```python
from build123d import *

# Parameters (mm, degrees)
BOSS_EXTRU_1_DEPTH      = 5
BOSS_EXTRU_2_DEPTH      = 80
ESQUISSE5_R             = 1.5
ENL_V_MAT_EXTRU_1_DEPTH = 85


with BuildPart() as part:
    # Esquisse1 → Boss.-Extru.1 (new body)
    with BuildSketch(Plane.XY):
        Polygon((90, 47.5), (80, 47.5), (80, 27.5), (90, 27.5), (90, 0), (80, 0), (80, 5), (60, 5), (60, 0), (30, 0), (30, 5), (10, 5), (10, 0), (0, 0), (0, 75), (10, 75), (10, 70), (30, 70), (30, 75), (60, 75), (60, 70), (80, 70), (80, 75), (90, 75), align=None)
    extrude(amount=BOSS_EXTRU_1_DEPTH)

    # Esquisse3 → Boss.-Extru.2 (add)
    with BuildSketch(Plane.ZY):
        Polygon((5, 18), (15, 18), (15, 5.25), (10, 5.25), (10, 13), (5, 13), align=None)
        Polygon((5, 62), (5, 57), (15, 57), (15, 69.75), (10, 69.75), (10, 62), align=None)
    extrude(amount=-BOSS_EXTRU_2_DEPTH)

    # Esquisse5 → Enlèv. mat.-Extru.1 (cut)
    with BuildSketch(Plane.ZY):
        with Locations((2.5, 2.5)):
            Circle(ESQUISSE5_R)
        with Locations((2.5, 72.5)):
            Circle(ESQUISSE5_R)
    extrude(amount=-ENL_V_MAT_EXTRU_1_DEPTH, mode=Mode.SUBTRACT)


solid = part.part
```
Geometry check sheet. Reference: the model listing, model coordinates, mm. A direction names the side the tool comes from. Give positions to 0.01 mm unless a question says otherwise; leave off trailing zeros. Loops run counter-clockwise (first coordinate to the right, second up) from the corner with the lowest first, then second, coordinate; pieces in that order, holes last. Notation, with made-up numbers: M 63,-27.5 L 96,-27.5 A22 cw 96,7.5 Z; hole C 28.5,72.25 d6. An arc over 180 degrees is marked long. Write item = value, one per line. Start each with the question number.
1. Draft check along Z on faces 6 (the face through (39, 63, 15)), 7 (the face through (85, 73, 2)), 8 (the face through (0, 37, 4)). Enter one of: +Z half, -Z half, draft (parallel to the pull), parting line (faces both ways), or undercut.
2. Section check C-C, the plane x = 6. Enter the section's corners in (y, z).
3. Go/stop test with flat-tipped pins: P1, Ø2.5, axis at x = 15.5, z = 2, coming from the -Y side; P2, Ø5, axis at x = 43, z = 8, coming from the +Y side; P3, Ø5, axis at x = 33, z = 11.5, coming from the -Y side. Record where each tip stops, or that it passes through.
4. Tool access check on faces 1 (the face through (39, 62, 8)), 2 (the face through (70, 70, 2)), 3 (the face through (39, 5.25, 13)), 4 (the face through (44.79, 73.765, 3.306)), 5 (the face through (70, 5, 2)). Record the directions out of +Z, -Z, +X, -X, +Y, -Y that give a thin tool (end or side, any length) a straight path to the whole face; none if there is none.
5. Section check B-B, the plane z = 7.5. Enter the section's corners in (x, y), plus the area to 3 significant figures.
6. Thickness scan on probe 1 along Y at (x, z) = (2.5, 2.5); probe 2 along Z at (x, y) = (57, 12); probe 3 along Y at (x, z) = (82.75, 2.5). Record the ranges inside material, lowest first.
7. Section check D-D, the plane y = 10. Enter the section's corners in (x, z), plus the area to 3 significant figures.
8. Section check A-A, the plane y = 2.5. Enter the section's corners in (x, z), plus the area to 3 significant figures.
Values follow:
q1.face_6 = +Z half
q1.face_7 = undercut
q1.face_8 = draft
q2.outline = M 0,0 L 75,0 L 75,5 L 62,5 L 62,10 L 69.75,10 L 69.75,15 L 57,15 L 57,5 L 18,5 L 18,15 L 5.25,15 L 5.25,10 L 13,10 L 13,5 L 0,5 Z; hole C 2.5,2.5 d3; hole C 72.5,2.5 d3
q3.P1 = 5
q3.P2 = 69.75
q3.P3 = 5.25
q4.face_1 = +X, -X, +Y
q4.face_2 = +Z, -Z, +Y
q4.face_3 = +Z, +X, -X, -Y
q4.face_4 = -X
q4.face_5 = +Z, -Z, -Y
q5.outline = M 0,13 L 80,13 L 80,18 L 0,18 Z; M 0,57 L 80,57 L 80,62 L 0,62 Z
q5.area = 800 mm^2
q6.probe_1 = 0 to 1, 4 to 71, 74 to 75
q6.probe_2 = 0 to 5, 10 to 15
q6.probe_3 = 0 to 1, 4 to 27.5, 47.5 to 71, 74 to 75
q7.outline = M 0,0 L 90,0 L 90,5 L 0,5 Z; M 0,10 L 80,10 L 80,15 L 0,15 Z
q7.area = 850 mm^2
q8.outline = M 0,0 L 10,0 L 10,1 L 0,1 Z; M 0,4 L 10,4 L 10,5 L 0,5 Z; M 30,0 L 60,0 L 60,1 L 30,1 Z; M 30,4 L 60,4 L 60,5 L 30,5 Z; M 80,0 L 90,0 L 90,5 L 80,5 L 80,4 L 85,4 L 85,1 L 80,1 Z
q8.area = 115 mm^2
